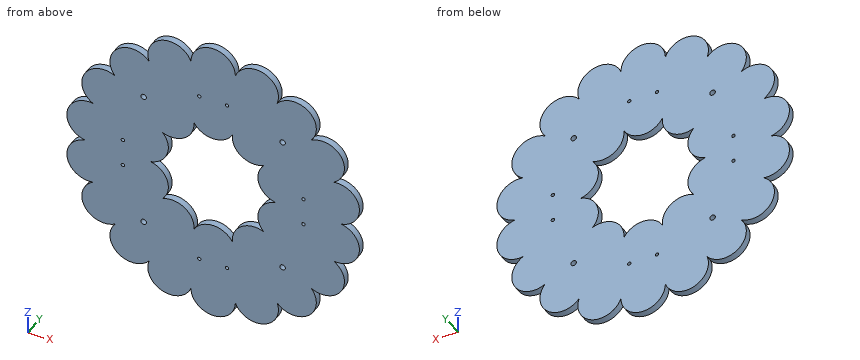
```python
from build123d import *

# Parameters (mm, degrees)
SKETCH1_R           = 115.202561211
SKETCH1_R_2         = 64.402561211
BOSS_EXTRUDE1_DEPTH = 6.35
SKETCH2_R           = 20.32
BOSS_EXTRUDE2_DEPTH = 6.35
SKETCH3_R           = 2.54
SKETCH3_R_2         = 1.524
CUT_EXTRUDE1_DEPTH  = 7.35


with BuildPart() as part:
    # Sketch1 → Boss-Extrude1 (new body)
    with BuildSketch(Plane(origin=(0, 0, 0), x_dir=(1, 0, 0), z_dir=(0, 1, 0))):
        Circle(SKETCH1_R)
        Circle(SKETCH1_R_2, mode=Mode.SUBTRACT)
    extrude(amount=BOSS_EXTRUDE1_DEPTH)

    # Sketch2 → Boss-Extrude2 (add)
    with BuildSketch(Plane(origin=(0, 6.35, 0), x_dir=(1, 0, 0), z_dir=(0, 1, 0))):
        with Locations((0, 64.402561211)):
            Circle(SKETCH2_R)
        with Locations((0, 115.202561211)):
            Circle(SKETCH2_R)
        with Locations((37.85487569, 52.102766501)):
            Circle(SKETCH2_R)
        with Locations((61.250475506, 19.901485895)):
            Circle(SKETCH2_R)
        with Locations((61.250475506, -19.901485895)):
            Circle(SKETCH2_R)
        with Locations((37.85487569, -52.102766501)):
            Circle(SKETCH2_R)
        with Locations((0, -64.402561211)):
            Circle(SKETCH2_R)
        with Locations((-37.85487569, -52.102766501)):
            Circle(SKETCH2_R)
        with Locations((-61.250475506, -19.901485895)):
            Circle(SKETCH2_R)
        with Locations((-61.250475506, 19.901485895)):
            Circle(SKETCH2_R)
        with Locations((-37.85487569, 52.102766501)):
            Circle(SKETCH2_R)
        with Locations((39.401596497, 108.254996665)):
            Circle(SKETCH2_R)
        with Locations((74.05077895, 88.250281849)):
            Circle(SKETCH2_R)
        with Locations((99.768344589, 57.601280605)):
            Circle(SKETCH2_R)
        with Locations((113.452375447, 20.004714817)):
            Circle(SKETCH2_R)
        with Locations((113.452375447, -20.004714817)):
            Circle(SKETCH2_R)
        with Locations((99.76834459, -57.601280605)):
            Circle(SKETCH2_R)
        with Locations((74.05077895, -88.250281849)):
            Circle(SKETCH2_R)
        with Locations((39.401596497, -108.254996665)):
            Circle(SKETCH2_R)
        with Locations((0, -115.202561211)):
            Circle(SKETCH2_R)
        with Locations((-39.401596497, -108.254996665)):
            Circle(SKETCH2_R)
        with Locations((-74.05077895, -88.250281849)):
            Circle(SKETCH2_R)
        with Locations((-99.768344589, -57.601280605)):
            Circle(SKETCH2_R)
        with Locations((-113.452375447, -20.004714817)):
            Circle(SKETCH2_R)
        with Locations((-113.452375447, 20.004714817)):
            Circle(SKETCH2_R)
        with Locations((-99.768344589, 57.601280605)):
            Circle(SKETCH2_R)
        with Locations((-74.05077895, 88.250281849)):
            Circle(SKETCH2_R)
        with Locations((-39.401596497, 108.254996665)):
            Circle(SKETCH2_R)
    extrude(amount=-BOSS_EXTRUDE2_DEPTH)

    # Sketch3 → Cut-Extrude1 (cut, through all)
    with BuildSketch(Plane(origin=(0, 6.35, 0), x_dir=(1, 0, 0), z_dir=(0, 1, 0))):
        with Locations((-63.5, 63.5)):
            Circle(SKETCH3_R)
        with Locations((-63.5, -63.5)):
            Circle(SKETCH3_R)
        with Locations((63.5, 63.5)):
            Circle(SKETCH3_R)
        with Locations((63.5, -63.5)):
            Circle(SKETCH3_R)
        with Locations((-12.7, 82.55)):
            Circle(SKETCH3_R_2)
        with Locations((12.7, 82.55)):
            Circle(SKETCH3_R_2)
        with Locations((82.55, 12.7)):
            Circle(SKETCH3_R_2)
        with Locations((82.55, -12.7)):
            Circle(SKETCH3_R_2)
        with Locations((12.7, -82.55)):
            Circle(SKETCH3_R_2)
        with Locations((-12.7, -82.55)):
            Circle(SKETCH3_R_2)
        with Locations((-82.55, -12.7)):
            Circle(SKETCH3_R_2)
        with Locations((-82.55, 12.7)):
            Circle(SKETCH3_R_2)
    extrude(amount=-CUT_EXTRUDE1_DEPTH, mode=Mode.SUBTRACT)


solid = part.part
```
The listing builds one solid part. Answer for the finished solid, in the listing's coordinates (mm). Coordinates: 2 decimals unless noted, no trailing zeros. Loops run counter-clockwise (first coordinate to the right, second up) from the corner with the lowest first, then second, coordinate; pieces in that order, holes last. Notation, with made-up numbers: (48, 89) -> (101, 89) arc R32 ccw to (101, 124) -> close; hole circle Ø4 at (-30.75, -24). An arc over 180 degrees is marked (long way). Use one line per item in the form item = value. Start each with the question number.
Item 1: Flat-ended cylindrical pins translate along their axes: pin 1 Ø1.5 at (x, y) = (-8.5, 1) entering from +Z; pin 2 Ø1.5 at (y, z) = (3.5, -72.5) entering from -X; pin 3 Ø1 at (y, z) = (4, -72.5) entering from +X. Find the tip coordinate at first contact, or state that the pin passes through.
Item 2: The part is cut by section A-A on x = 34. Determine the outline of the cut face in (y, z).
Item 3: The part is cut by section B-B on y = 4.75. Count the separate pieces of the cut face and the enclosed holes in it, then the cut area to 3 significant figures.
Item 4: Consider L1, parallel to Z at x = 63.5, y = 4.75; L2, parallel to X at y = 5.75, z = -45.5; L3, parallel to X at y = 3.75, z = 12.7. Determine where each line is inside the solid, lowest interval first. Write a range as [from, to].
Answer key:
q1.pin_1 = 133.99
q1.pin_2 = -114.35
q1.pin_3 = 114.11
q2.outline = (0, -127.84) -> (6.35, -127.84) -> (6.35, -32.15) -> (0, -32.15) -> close; (0, 32.15) -> (6.35, 32.15) -> (6.35, 127.84) -> (0, 127.84) -> close
q3.separate_pieces = 1
q3.enclosed_holes = 13
q3.area = 46,600 mm2
q4.L1 = [-105.62, -66.04], [-60.96, 60.96], [66.04, 105.62]
q4.L2 = [-116.09, -18.64], [-7.46, 7.46], [18.64, 116.09]
q4.L3 = [-132.41, -84.07], [-81.03, -42.25], [42.25, 81.03], [84.07, 132.41]
